```python
from build123d import *

# Parameters (mm, degrees)
F_23_0_23_DIAMETER_HOLE2_D = 23
M5_CLEARANCE_HOLE1_D       = 5.64
M5_CLEARANCE_HOLE1_DEPTH   = 10
M25_CLEARANCE_HOLE1_D      = 28.2


with BuildPart() as part:
    # Sketch1 → Revolve1 (revolve)
    with BuildSketch(Plane(origin=(0, 0, 0), x_dir=(-1, 0, 0), z_dir=(0, 0, -1))):
        with BuildLine():
            Line((0, -21.28), (-47, -21.28))
            add(Edge.make_bspline(
                [(-47, -21.28), (-48.103397798, -21.28), (-50.355208609, -21.119817001), (-53.414331373, -20.453461244), (-56.243773206, -19.439198841), (-59.638625381, -17.760520516), (-63.24918477, -15.301778213), (-66.920694033, -12.332831089), (-70.220914899, -9.726996026), (-72.788397394, -8.094435047), (-74.823949114, -7.162885506), (-76.366758302, -6.651929985), (-77.75784267, -6.37664197), (-78.927463, -6.261355146), (-79.581421905, -6.24), (-79.9, -6.24)],
                knots=[0, 0, 0, 0, 0.0625, 0.125, 0.1875, 0.25, 0.375, 0.5, 0.625, 0.75, 0.8125, 0.875, 0.9375, 0.96875, 1, 1, 1, 1], degree=3))
            Line((-79.9, -6.24), (-109.626011544, -6.24))
            Line((-109.626011544, -6.24), (-109.626011544, 3.76))
            Line((-109.626011544, 3.76), (-79.9, 3.76))
            add(Edge.make_bspline(
                [(-47, -11.28), (-47.323760623, -11.28), (-47.9824274, -11.256801184), (-49.205881481, -11.125337538), (-50.652473039, -10.813460463), (-52.303634488, -10.223599604), (-54.465904258, -9.163050099), (-57.16913982, -7.350711887), (-60.559773273, -4.61985368), (-64.271682561, -1.670850737), (-67.847161888, 0.63981733), (-71.12599799, 2.151104958), (-73.810430606, 3.042514571), (-76.243250574, 3.525131309), (-78.291888688, 3.725497683), (-79.368008784, 3.76), (-79.9, 3.76)],
                knots=[0, 0, 0, 0, 0.03125, 0.0625, 0.125, 0.1875, 0.25, 0.375, 0.5, 0.625, 0.75, 0.8125, 0.875, 0.9375, 0.96875, 1, 1, 1, 1], degree=3))
            Line((-47, -11.28), (0, -11.28))
            Line((0, -11.28), (0, -21.28))
        make_face()
    revolve(axis=Axis((0, -15.043324423, 0), (0, 1, 0)))

    # Ø23.0 (23) Diameter Hole2 (through all)
    with Locations(Plane(origin=(0, 3.76, 0), x_dir=(1, 0, 0), z_dir=(0, 1, 0))):
        with Locations((-92.997954647, 53.69239415), (92.997954647, -53.69239415), (92.997954647, 53.69239415), (0, 107.3847883), (-92.997954647, -53.69239415), (0, -107.3847883)):
            Hole(F_23_0_23_DIAMETER_HOLE2_D / 2)

    # M5 Clearance Hole1
    with Locations(Plane(origin=(0, -11.28, 0), x_dir=(1, 0, 0), z_dir=(0, 1, 0))):
        with Locations((-32.562555182, 18.8), (0, 37.6), (32.562555182, 18.8), (32.562555182, -18.8), (0, -37.6), (-32.562555182, -18.8)):
            Hole(M5_CLEARANCE_HOLE1_D / 2, depth=M5_CLEARANCE_HOLE1_DEPTH)

    # M25 Clearance Hole1 (through all)
    with Locations(Plane(origin=(0, -11.28, 0), x_dir=(1, 0, 0), z_dir=(0, 1, 0))):
        with Locations((0, 0)):
            Hole(M25_CLEARANCE_HOLE1_D / 2)


solid = part.part
```
Verification items for the finished model (mm, model axes). A direction names the side the tool comes from. Coordinates: 2 decimals unless noted, no trailing zeros. Answer in a Markdown table with one row per item.
1) Draft check along Z on faces 1 (the face through (109.624, -1.17, 0.644)), 2 (the face through (-54.25, -1.17, -95.26)), 3 (the face through (-1, 3.76, -81)), 4 (the face through (34.8, -16.35, -17.084)). Enter one of: released by +Z, released by -Z, zero draft, split by the parting line, or undercut.
The answers:
| item | result |
|---|---|
| face 1 | split by the parting line |
| face 2 | released by -Z |
| face 3 | zero draft |
| face 4 | undercut |
2) Depth check by flat-ended pin: P1, Ø8, axis at x = -77.5, z = -63, coming from the -Y side; P2, Ø2, axis at x = -56.5, y = -1, coming from the -Z side; P3, Ø6, axis at x = 2.5, z = -14.5, coming from the +Y side. Enter the tip coordinate at first touch or a pass-through.
The answers:
| item | result |
|---|---|
| P1 | stops at y = -6.24 |
| P2 | stops at z = -94.54 |
| P3 | stops at y = -11.28 |
3) Section check A-A (x = 0). Give the number of separate pieces and of enclosed holes in the cut face, and give its area (3 significant figures).
The answers:
| item | result |
|---|---|
| separate pieces | 4 |
| enclosed holes | 0 |
| area | 1,600 mm2 |
4) Access from +Z, -Z, +X, -X, +Y, -Y to the whole of each face (thin tool, end or side, straight path). Record for faces 5 (the face through (1, -6.24, -81)), 6 (the face through (-6.506, -16.35, 12.509)), 7 (the face through (10, -11.28, -11)).
The answers:
| item | result |
|---|---|
| face 5 | -Y |
| face 6 | +Y, -Y |
| face 7 | +Y |
5) Scan lines: line 1 along X through (y, z) = (-13.75, -18.8); line 2 along Z through (x, y) = (0, -18.5); line 3 along X through (y, z) = (-12, 18). Record each from-to range of solid material in increasing order. Write a range as from..to.
The answers:
| item | result |
|---|---|
| line 1 | x = -62.39..-35.38, -29.74..29.74, 35.38..62.39 |
| line 2 | z = -58.1..-40.42, -34.78..-14.1, 14.1..34.78, 40.42..58.1 |
| line 3 | x = -64.9..-35.27, -29.86..29.86, 35.27..64.9 |
